Source: three-view drawing plus pictorial views. Frame: mm from the lowest corner of the part. Give positions to 0.01 mm unless a question says otherwise; leave off trailing zeros. Order: outer loops, then holes, each group sorted by start corner. A loop starts at its lowest first (then second) coordinate and runs counter-clockwise, first axis right, second up. Notation, with made-up numbers: (15.5, -26.5) -> (66.5, -26.5) arc R23 ccw to (66.5, -7.5) -> close; hole circle Ø3 at (86.5, 65). An arc over 180 degrees is marked (long way). One line per question, with ' | ' between items.
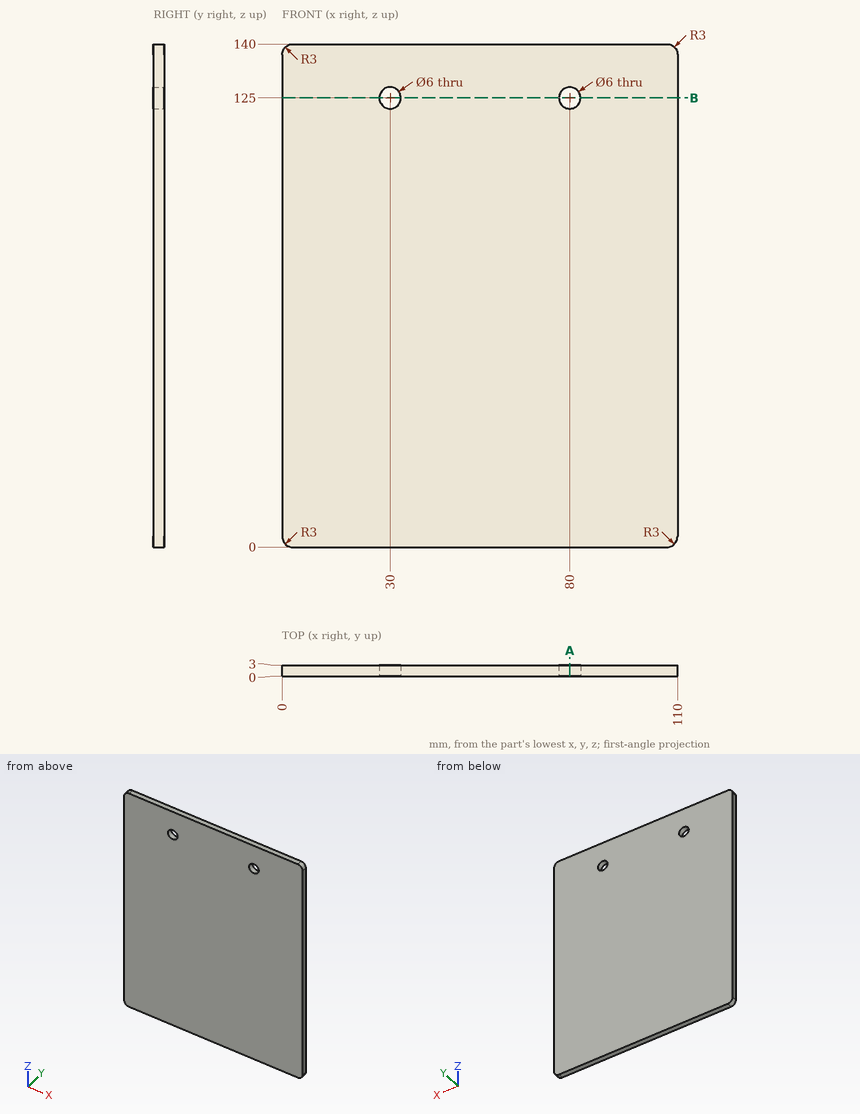
1) Contact query for a flat-ended pin moving along its axis: pin 1 Ø1 at (x, z) = (65.5, 101) entering from -Y. Output: stop coordinate, or through.
Check result:
pin 1: stops at y = 0
2) Section B-B on z = 125. Return loops of the section in (x, y).
Check result:
outline: (0, 0) -> (27, 0) -> (27, 3) -> (0, 3) -> close; (33, 0) -> (77, 0) -> (77, 3) -> (33, 3) -> close; (83, 0) -> (110, 0) -> (110, 3) -> (83, 3) -> close
3) Section A-A on x = 80. Return loops of the section in (y, z), plus the area to 3 significant figures.
Check result:
outline: (0, 0) -> (3, 0) -> (3, 122) -> (0, 122) -> close; (0, 128) -> (3, 128) -> (3, 140) -> (0, 140) -> close | area: 402 mm^2
4) Material intervals for probe 1 along X at (y, z) = (2.45, 125); probe 2 along Z at (x, y) = (80, 1.05); probe 3 along Z at (x, y) = (31, 0.45), sorted ascending. Write a range as from..to.
Check result:
probe 1: x = 0..27, 33..77, 83..110 | probe 2: z = 0..122, 128..140 | probe 3: z = 0..122.17, 127.83..140
